from build123d import *

# Parameters (mm, degrees)
SKETCH1_W               = 25.4
SKETCH1_H               = 25.4
SKETCH1_W_2             = 20.32
SKETCH1_H_2             = 20.32
BOSS_EXTRUDE1_DEPTH     = 241.3
CUT_EXTRUDE1_DEPTH      = 243.965306165
CUT_EXTRUDE1_DEPTH_BACK = 243.965306165
SKETCH2_R               = 5
CUT_EXTRUDE3_DEPTH      = 243.965306165
CUT_EXTRUDE3_DEPTH_BACK = 243.965306165
SKETCH5_R               = 2.5


with BuildPart() as part:
    # Sketch1 → Boss-Extrude1 (new, symmetric)
    with BuildSketch(Plane.XY):
        Rectangle(SKETCH1_W, SKETCH1_H)
        Rectangle(SKETCH1_W_2, SKETCH1_H_2, mode=Mode.SUBTRACT)
    extrude(amount=BOSS_EXTRUDE1_DEPTH, both=True)

    # Sketch2 → Cut-Extrude1 (cut, two sides: drawn at the far end of the back side and taken through both)
    with BuildSketch(Plane.ZY.offset(12.7).offset(-CUT_EXTRUDE1_DEPTH_BACK)):
        with Locations(Location((-212.1, 3.81, 0), (0, 0, 270))):
            Circle(SKETCH2_R)
        with Locations(Location((-160.1, 3.81, 0), (0, 0, 270))):
            Circle(SKETCH2_R)
    extrude(amount=CUT_EXTRUDE1_DEPTH + CUT_EXTRUDE1_DEPTH_BACK, mode=Mode.SUBTRACT)

    # Sketch5 → Cut-Extrude3 (cut, two sides: drawn at the far end of the back side and taken through both)
    with BuildSketch(Plane.ZY.offset(12.7).offset(-CUT_EXTRUDE3_DEPTH_BACK)):
        with Locations(Location((-194.85, 0, 0), (0, 0, 270))):
            Circle(SKETCH5_R)
        with Locations(Location((-177.35, 0, 0), (0, 0, 270))):
            Circle(SKETCH5_R)
    extrude(amount=CUT_EXTRUDE3_DEPTH + CUT_EXTRUDE3_DEPTH_BACK, mode=Mode.SUBTRACT)


solid = part.part
Check sheet for the modelled part. Datum: model origin and axes. Units: mm. A direction names the side the tool comes from. Round coordinates to 2 decimals unless told otherwise and drop trailing zeros. Order: outer loops, then holes, each group sorted by start corner. A loop starts at its lowest first (then second) coordinate and runs counter-clockwise, first axis right, second up. Notation, with made-up numbers: M -22.75,36.5 L 15.25,36.5 A26 ccw 15.25,74.5 Z; hole C 36.25,39 d4. An arc over 180 degrees is marked long. One line per item, written item: value. Start each with the question number.
1. Section check B-B on x = 5.5. Enter the section's corners in (y, z), and give its area (3 significant figures).
2. Scan lines: line 1 along Z through (x, y) = (-11.05, 3.81); line 2 along X through (y, z) = (-9.75, 52); line 3 along Y through (x, z) = (-10.65, -194.85). Record each from-to range of solid material in increasing order.
3. Section check C-C on z = 63. Enter the section's corners in (x, y).
4. Section check A-A on z = -212.1. Enter the section's corners in (x, y), and give its area (3 significant figures).
5. Access from +Z, -Z, +X, -X, +Y, -Y to the whole of each face (thin tool, end or side, straight path). Record for faces 5 (the flat face through (0, -10.16, 3)), 6 (the flat face through (0, 12.7, 3)).
6. Release check for a two-part mould opening along Z. For faces 1 (the cylindrical face through (-11.412, 4.461, -207.143)), 2 (the flat face through (11, 0, 241.3)), 3 (the flat face through (-12.7, 0, 3)), 4 (the cylindrical face through (11.448, 4.461, -207.143)) record: released by +Z, released by -Z, zero draft, split by the parting line, or undercut.
Results found:
1. outline: M -12.7,-241.3 L -10.16,-241.3 L -10.16,241.3 L -12.7,241.3 Z; M 10.16,-241.3 L 12.7,-241.3 L 12.7,241.3 L 10.16,241.3 Z
1. area: 2,450 mm^2
2. line 1: -241.3 to -217.1, -207.1 to -165.1, -155.1 to 241.3
2. line 2: -12.7 to -10.16, 10.16 to 12.7
2. line 3: -12.7 to -2.5, 2.5 to 12.7
3. outline: M -12.7,-12.7 L 12.7,-12.7 L 12.7,12.7 L -12.7,12.7 Z; hole M -10.16,-10.16 L 10.16,-10.16 L 10.16,10.16 L -10.16,10.16 Z
4. outline: M -12.7,-12.7 L 12.7,-12.7 L 12.7,-1.19 L 10.16,-1.19 L 10.16,-10.16 L -10.16,-10.16 L -10.16,-1.19 L -12.7,-1.19 Z; M -12.7,8.81 L -10.16,8.81 L -10.16,10.16 L 10.16,10.16 L 10.16,8.81 L 12.7,8.81 L 12.7,12.7 L -12.7,12.7 Z
4. area: 181 mm^2
5. face 5: +Z, -Z
5. face 6: +Z, -Z, +X, -X, +Y
6. face 1: undercut
6. face 2: released by +Z
6. face 3: zero draft
6. face 4: undercut
